```python
from build123d import *

# Parameters (mm, degrees)
BOX001_W               = 20
BOX001_H               = 7.07
BOX001_DEPTH           = 7.07
BOX001_PLACEMENT_ANGLE = 44.999934
BOX_W                  = 20
BOX_H                  = 10
BOX_DEPTH              = 10


with BuildPart() as base:
    # Box001 → Box001 (new body)
    with BuildSketch(Plane.XY):
        with Locations((10, 3.535)):
            Rectangle(BOX001_W, BOX001_H)
    extrude(amount=BOX001_DEPTH)


with BuildPart() as base_1:
    # Box001 placement: moved
    add(base.part.moved(Location((-10, -5, 10))).rotate(Axis((-10, -5, 10), (-1, 0, 0)), BOX001_PLACEMENT_ANGLE))


with BuildPart() as fusion:
    # Box → Box (new body)
    with BuildSketch(Plane(origin=(-10, -5, 0), x_dir=(1, 0, 0), z_dir=(0, 0, 1))):
        with Locations((10, 5)):
            Rectangle(BOX_W, BOX_H)
    extrude(amount=BOX_DEPTH)

    # Fusion: union Base
    add(base_1.part)


solid = fusion.part
```
Geometry: final body of the model. Coordinates: model frame, mm. Round coordinates to 2 decimals unless told otherwise and drop trailing zeros. Loops run counter-clockwise (first coordinate to the right, second up) from the corner with the lowest first, then second, coordinate; pieces in that order, holes last.
Item 1: Section B-B, the plane y = 4. Output: boundary loops of the cut face in (x, z).
Checked values:
outline: (-10, 0) - (10, 0) - (10, 11) - (-10, 11) - close
Item 2: Contact query for flat-ended pins moving along their axis: P1, Ø5, axis at x = -6, y = -0.5, coming from the +Z side; P2, Ø5, axis at x = 6, z = 11, coming from the +Y side; P3, Ø5, axis at x = 6.5, y = -3, coming from the +Z side. Output: stop coordinate, or through.
Checked values:
P1: stops at z = 15
P2: stops at y = 5
P3: stops at z = 14.5
Item 3: Line query: L1, parallel to Z at x = 3, y = 1.25; L2, parallel to Z at x = 3.25, y = 0.75; L3, parallel to Y at x = -0.5, z = 12.75. Output: solid intervals per line, ascending.
Checked values:
L1: z = 0 to 13.75
L2: z = 0 to 14.25
L3: y = -2.25 to 2.25
Item 4: Section C-C, the plane z = 10.25. Output: boundary loops of the cut face in (x, y), plus the area to 3 significant figures.
Checked values:
outline: (-10, -4.75) - (10, -4.75) - (10, 4.75) - (-10, 4.75) - close
area: 190 mm2
